For this review, take the finished solid that the model builds, in its own axes (mm). A direction names the side the tool comes from. Coordinates: 2 decimals unless noted, no trailing zeros. Loops run counter-clockwise (first coordinate to the right, second up) from the corner with the lowest first, then second, coordinate; pieces in that order, holes last. Notation, with made-up numbers: M -32.75,3 L -2.75,3 A9 cw -2.75,12 Z; hole C -26,68 d10. An arc over 180 degrees is marked long. Write item = value, one per line.
from build123d import *

# Parameters (mm, degrees)
F0_W      = 264
F0_H      = 134
F1_DEPTH  = 62
F3_DEPTH  = 150
F7_START  = -33.8
F7_DEPTH  = 66.4
F8_T      = -2
F9_R      = 1.75
F10_DEPTH = 134.001
F11_R     = 1.75
F12_DEPTH = 25
F14_START = -13
F13_W     = 15.5
F13_H     = 15.5
F13_R     = 1.75
F14_DEPTH = 6


# Not quite as in the source:
# - a feature of the source that left no trace in its solid (it failed there, or was rolled back) is left out


with BuildPart() as f1:
    # F0 (on Top) → F1 (new body, symmetric)
    with BuildSketch(Plane.XY):
        Rectangle(F0_W, F0_H)
    extrude(amount=F1_DEPTH, both=True)

    # F2 (on face) → F3 (cut)
    with BuildSketch(Plane.XZ.offset(67)):
        with BuildLine():
            ThreePointArc((-132, -62), (-95.6812408671, 25.6812408671), (-8, 62))
            Line((-8, 62), (-132, 62))
            Line((-132, 62), (-132, -62))
        make_face()
    extrude(amount=-F3_DEPTH, mode=Mode.SUBTRACT)

    # F6 (on face) → F7 (cut)
    with BuildSketch(Plane.XZ.offset(67).offset(F7_START)):
        Polygon((-105.1785842524, 21.3899467149), (-98.1075164406, 14.318878903), (-86.8645186197, 25.5618767239), (-93.9355864316, 32.6329445358), align=None)
    extrude(amount=-F7_DEPTH, mode=Mode.SUBTRACT)

    # F8
    f8_openings = [f1.faces().sort_by_distance(p)[0] for p in [
        (132, 0, 0),
    ]]
    offset(amount=F8_T, openings=f8_openings, kind=Kind.INTERSECTION)

    # F9 (on face) → F10 (cut, through all)
    with BuildSketch(Plane.XZ.offset(67)):
        with Locations((102, 12)):
            Circle(F9_R)
        with Locations((2, 12)):
            Circle(F9_R)
    extrude(amount=-F10_DEPTH, mode=Mode.SUBTRACT)

    # F11 (on face) → F12 (cut)
    with BuildSketch(Plane.XZ.offset(67)):
        with BuildLine():
            ThreePointArc((-26.79829216, 31.0818016827), (-28.2627582541, 34.6173355886), (-31.79829216, 36.0818016827))
            Line((-31.79829216, 36.0818016827), (-50.79829216, 36.0818016827))
            ThreePointArc((-50.79829216, 36.0818016827), (-54.333826066, 34.6173355886), (-55.79829216, 31.0818016827))
            Line((-55.79829216, 31.0818016827), (-55.79829216, -11.9181983173))
            Line((-55.79829216, -11.9181983173), (-26.79829216, -11.9181983173))
            Line((-26.79829216, -11.9181983173), (-26.79829216, 31.0818016827))
        make_face()
        with Locations((-61.29829216, 12.0818016827)):
            Circle(F11_R)
        with Locations((-21.29829216, 12.0818016827)):
            Circle(F11_R)
    extrude(amount=-F12_DEPTH, mode=Mode.SUBTRACT)

    # F13 (on face) → F14 (join)
    with BuildSketch(Plane.YZ.offset(132).offset(F14_START)):
        with Locations((-57.25, 52.25)):
            Rectangle(F13_W, F13_H)
        with Locations((-57.25, 52.25)):
            Circle(F13_R, mode=Mode.SUBTRACT)
        with Locations((57.25, 52.25)):
            Rectangle(F13_W, F13_H)
        with Locations((57.25, 52.25)):
            Circle(F13_R, mode=Mode.SUBTRACT)
        with Locations((57.25, -52.25)):
            Rectangle(F13_W, F13_H)
        with Locations((57.25, -52.25)):
            Circle(F13_R, mode=Mode.SUBTRACT)
        with Locations((-57.25, -52.25)):
            Rectangle(F13_W, F13_H)
        with Locations((-57.25, -52.25)):
            Circle(F13_R, mode=Mode.SUBTRACT)
    extrude(amount=-F14_DEPTH)


solid = f1.part
Q1. Add section D-D (z = -34.5). Write out the cut boundary in (x, y), and give its area (3 significant figures).
Solved:
outline = M -128.91,-67 L 132,-67 L 132,-65 L -126.86,-65 L -126.86,65 L 132,65 L 132,67 L -128.91,67 Z
area = 1,310 mm²
Q2. For line 1 along Y through (x, z) = (116, -52); line 2 along Z through (x, y) = (116.9, 57.25); line 3 along Z through (x, y) = (32.5, -51), list the stretches that pass through material, from the lowest coordinate up.
Solved:
line_1 = -67 to -58.98, -55.52 to -49.5, 49.5 to 55.52, 58.98 to 67
line_2 = -62 to -54, -50.5 to -44.5, 44.5 to 50.5, 54 to 62
line_3 = -62 to -60, 60 to 62
Q3. Add section A-A (x = 41.5). Write out the cut boundary in (y, z), and give its area (3 significant figures).
Solved:
outline = M -67,-62 L 67,-62 L 67,62 L -67,62 Z; hole M -65,-60 L 65,-60 L 65,60 L -65,60 Z
area = 1,020 mm²
Q4. Draft analysis for pull direction X (two halves, no side actions). For faces 1 (the face through (-93, 35.2, 21)), 2 (the face through (-95, -33.2, 22)), 3 (the face through (-110.35, -0.94, 8)), 4 (the face through (-28.224, -66.014, 34.578)), state which applies: +X half, -X half, draft (parallel to the pull), parting line (faces both ways), or undercut.
Solved:
face_1 = draft
face_2 = undercut
face_3 = -X half
face_4 = undercut
Q5. Add section B-B (z = 5). Write out the cut boundary in (x, y).
Solved:
outline = M -112.34,-67 L -55.8,-67 L -55.8,-65 L -109.96,-65 L -109.96,65 L 132,65 L 132,67 L -112.34,67 Z; M -26.8,-67 L 132,-67 L 132,-65 L -26.8,-65 Z
Q6. Machinability: for faces 5 (the face through (61, 1, 62)), 6 (the face through (-1, 65, 1)), 7 (the face through (116, -49.5, -52)), which of the approach directions +Z, -Z, +X, -X, +Y, -Y give a long, thin tool a straight path to every point of the face, cutting with its end or side? Answer none if there is none.
Solved:
face_5 = +Z, +X, -X, +Y, -Y
face_6 = none
face_7 = +X
Q7. For pin 1 Ø6 at (y, z) = (52.5, 34.5) entering from +X; pin 2 Ø4.5 at (y, z) = (54, 50) entering from +X; pin 3 Ø3 at (y, z) = (-57.25, 52.25) entering from -X; pin 4 Ø2 at (x, z) = (2, 12) entering from -Y, all flat-tipped, find the tip position at first contact; note any pin that passes through.
Solved:
pin_1 = -78.6
pin_2 = 119
pin_3 = -59.61
pin_4 = through
Q8. Add section C-C (y = -26). Write out the cut boundary in (x, z).
Solved:
outline = M -132,-62 L 132,-62 L 132,-60 L -129.98,-60 A122 cw -102.17,15.56 L -98.11,11.49 L -84.04,25.56 L -88.31,29.84 A122 cw -8,60 L 132,60 L 132,62 L -8,62 A124 ccw -91.22,29.92 L -86.86,25.56 L -98.11,14.32 L -102.3,18.52 A124 ccw Z
